Check sheet for the modelled part. Datum: model origin and axes. Units: mm. Face numbers are marked on the shaded views. A direction names the side the tool comes from. Round coordinates to 2 decimals unless told otherwise and drop trailing zeros. Write each loop counter-clockwise with the first axis right and the second up, starting at its lowest first coordinate (ties: lowest second). Pieces come first, ordered by that corner, then holes. Notation, with made-up numbers: (57.5, 32) - (61.5, 32) arc R29 ccw to (61.5, 61) - close; hole circle Ø1 at (-34.75, 61). An arc over 180 degrees is marked (long way). Answer as a JSON object with one key per item and string values. Group by question number.
Item 1: Thickness scan on line 1 (Z direction, x = 69, y = 6.75); line 2 (X direction, y = 5.75, z = -8); line 3 (X direction, y = 0.5, z = 5.5). Record the ranges inside material, lowest first.
Item 2: Set-up check for the marked faces 1, 2, 3 and 4: record each of +Z, -Z, +X, -X, +Y, -Y from which the full face is reachable in a straight line by a thin tool's end or side.
Item 3: Sectioned sample at D-D on z = -32. Record the boundary of the cut face in (x, y), plus the area to 3 significant figures.
Item 4: Sectioned sample at C-C on y = 1.5. Count the separate pieces of the cut face and the enclosed holes in it, plus the area to 3 significant figures.
Item 5: Gauge pin test, flat ends, axial feed: P1, Ø4.5, axis at x = 73.5, z = 5.5, coming from the +Y side; P2, Ø4, axis at x = 60, y = 3.5, coming from the +Z side; P3, Ø2, axis at y = 3, z = 17, coming from the -X side; P4, Ø3.5, axis at x = 90.01, z = -24.99, coming from the +Y side. Record the tip position at first contact, or that the pin passes through.
Item 6: Sectioned sample at B-B on x = 60. Record the boundary of the cut face in (y, z), plus the area to 3 significant figures.
Item 7: Sectioned sample at A-A on z = 16. Record the boundary of the cut face in (x, y), plus the area to 3 significant figures.
Item 8: Release check for a two-part mould opening along Z. For the marked faces 5, 6 and 7 record: pulls with the +Z half, pulls with the -Z half, needs draft (parallel to the pull), parting line crosses it, or undercut.
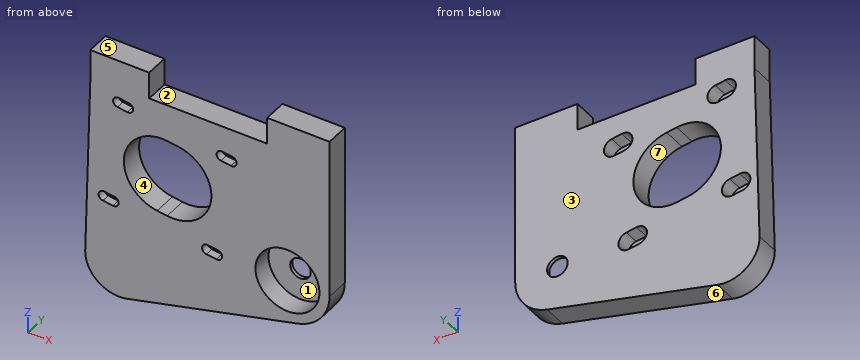
```python
from build123d import *

# Parameters (mm, degrees)
SKETCH2_R           = 3.05
BOSS_EXTRUDE1_DEPTH = 7
SKETCH2_7_R         = 9.5
SKETCH2_7_R_2       = 3.05
CUT_EXTRUDE1_DEPTH  = 6
CUT_EXTRUDE2_START  = 7
CUT_EXTRUDE2_DEPTH  = 4.5


with BuildPart() as part:
    # Sketch2 → Boss-Extrude1 (new body)
    with BuildSketch(Plane(origin=(0, 0, 0), x_dir=(1, 0, 0), z_dir=(0, 1, 0))):
        with BuildLine():
            Line((102.512048312, 24.992099408), (102.512048312, -23.007900592))
            Line((102.512048312, -23.007900592), (84.012048312, -23.007900592))
            Line((84.012048312, -23.007900592), (84.012048312, -15.007900592))
            Line((84.012048312, -15.007900592), (49.012048312, -15.007900592))
            Line((49.012048312, -15.007900592), (49.012048312, -23.007900592))
            Line((49.012048312, -23.007900592), (31.512048312, -23.007900592))
            Line((31.512048312, -23.007900592), (31.512048312, -13.007900592))
            Line((31.512048312, -13.007900592), (30.016072392, 39.708435169))
            ThreePointArc((30.016072392, 39.708435169), (33.741164308, 47.78158038), (42.423514406, 49.696986387))
            Line((42.423514406, 49.696986387), (93.026380929, 37.123208132))
            ThreePointArc((93.026380929, 37.123208132), (99.859107713, 32.691802074), (102.512048312, 24.992099408))
        make_face()
        with Locations(Location((90.012048312, 24.992099408, 0), (0, 0, 270))):
            Circle(SKETCH2_R, mode=Mode.SUBTRACT)
        with BuildLine():
            Line((51.378851017, 18.833843692), (54.349655223, 19.251362995))
            ThreePointArc((54.349655223, 19.251362995), (67.338228674, 9.463770865), (57.550636545, -3.524802586))
            Line((57.550636545, -3.524802586), (54.579832339, -3.942321889))
            ThreePointArc((54.579832339, -3.942321889), (41.591258887, 5.84527024), (51.378851017, 18.833843692))
        make_face(mode=Mode.SUBTRACT)
        with BuildLine():
            Line((65.962554027, 26.437501135), (68.933358233, 26.855020438))
            ThreePointArc((68.933358233, 26.855020438), (70.627519988, 25.578377986), (69.350877536, 23.884216232))
            Line((69.350877536, 23.884216232), (66.38007333, 23.466696929))
            ThreePointArc((66.38007333, 23.466696929), (64.685911575, 24.74333938), (65.962554027, 26.437501135))
        make_face(mode=Mode.SUBTRACT)
        with BuildLine():
            Line((70.694439459, -7.231613202), (73.665243666, -6.814093899))
            ThreePointArc((73.665243666, -6.814093899), (74.941886117, -5.119932145), (73.247724363, -3.843289693))
            Line((73.247724363, -3.843289693), (70.276920157, -4.260808996))
            ThreePointArc((70.276920157, -4.260808996), (69.000277705, -5.954970751), (70.694439459, -7.231613202))
        make_face(mode=Mode.SUBTRACT)
        with BuildLine():
            Line((42.966933535, -11.128460029), (39.996129329, -11.545979332))
            ThreePointArc((39.996129329, -11.545979332), (38.301967574, -10.26933688), (39.578610026, -8.575175126))
            Line((39.578610026, -8.575175126), (42.549414232, -8.157655823))
            ThreePointArc((42.549414232, -8.157655823), (44.243575986, -9.434298275), (42.966933535, -11.128460029))
        make_face(mode=Mode.SUBTRACT)
        with BuildLine():
            Line((38.235048102, 22.540654308), (35.264243896, 22.123135005))
            ThreePointArc((35.264243896, 22.123135005), (33.987601444, 20.428973251), (35.681763199, 19.152330799))
            Line((35.681763199, 19.152330799), (38.652567405, 19.569850102))
            ThreePointArc((38.652567405, 19.569850102), (39.929209857, 21.264011856), (38.235048102, 22.540654308))
        make_face(mode=Mode.SUBTRACT)
    extrude(amount=BOSS_EXTRUDE1_DEPTH)

    # Sketch2<7> → Cut-Extrude1 (cut)
    with BuildSketch(Plane(origin=(0, 0, 0), x_dir=(1, 0, 0), z_dir=(0, 1, 0))):
        with Locations(Location((90.012048312, 24.992099408, 0), (0, 0, 270))):
            Circle(SKETCH2_7_R)
        with Locations(Location((90.012048312, 24.992099408, 0), (0, 0, 270))):
            Circle(SKETCH2_7_R_2, mode=Mode.SUBTRACT)
    extrude(amount=CUT_EXTRUDE1_DEPTH, mode=Mode.SUBTRACT)

    # Sketch2<8> → Cut-Extrude2 (cut)
    with BuildSketch(Plane(origin=(0, 0, 0), x_dir=(1, 0, 0), z_dir=(0, 1, 0)).offset(CUT_EXTRUDE2_START)):
        with BuildLine():
            Line((65.788587651, 27.675336221), (68.759391857, 28.092855524))
            ThreePointArc((68.759391857, 28.092855524), (71.865355074, 25.752344362), (69.524843912, 22.646381146))
            Line((69.524843912, 22.646381146), (66.554039706, 22.228861843))
            ThreePointArc((66.554039706, 22.228861843), (63.448076489, 24.569373004), (65.788587651, 27.675336221))
        make_face()
        with BuildLine():
            Line((70.868405836, -8.469448288), (73.839210042, -8.051928985))
            ThreePointArc((73.839210042, -8.051928985), (76.179721203, -4.945965769), (73.073757987, -2.605454607))
            Line((73.073757987, -2.605454607), (70.10295378, -3.02297391))
            ThreePointArc((70.10295378, -3.02297391), (67.762442619, -6.128937127), (70.868405836, -8.469448288))
        make_face()
        with BuildLine():
            Line((38.061081726, 23.778489394), (35.09027752, 23.360970091))
            ThreePointArc((35.09027752, 23.360970091), (32.749766358, 20.255006874), (35.855729575, 17.914495713))
            Line((35.855729575, 17.914495713), (38.826533781, 18.332015016))
            ThreePointArc((38.826533781, 18.332015016), (41.167044943, 21.437978232), (38.061081726, 23.778489394))
        make_face()
        with BuildLine():
            Line((42.375447856, -6.919820737), (39.404643649, -7.33734004))
            ThreePointArc((39.404643649, -7.33734004), (37.064132488, -10.443303257), (40.170095705, -12.783814418))
            Line((40.170095705, -12.783814418), (43.140899911, -12.366295115))
            ThreePointArc((43.140899911, -12.366295115), (45.481411072, -9.260331898), (42.375447856, -6.919820737))
        make_face()
    extrude(amount=-CUT_EXTRUDE2_DEPTH, mode=Mode.SUBTRACT)


solid = part.part
```
Completed:
{
 "1": {"line 1": "-43.09 to -28.12, -22.57 to 3.43, 8.06 to 15.01", "line 2": "30.92 to 41.49, 67.45 to 102.51", "line 3": "31.3 to 69.01, 74.95 to 102.51"},
 "2": {"face 1": "-Y", "face 2": "+Z, +Y, -Y", "face 3": "+Z, -Z, +X, -X, +Y", "face 4": "+Y, -Y"},
 "3": {"outline": "(30.23, 0) - (83.6, 0) - (83.6, 6) - (96.43, 6) - (96.43, 0) - (100.36, 0) - (100.36, 7) - (30.23, 7) - close", "area": "414 mm²"},
 "4": {"separate pieces": "1", "enclosed holes": "6", "area": "3,620 mm²"},
 "5": {"P1": "y = 2.5", "P2": "z = 15.01", "P3": "x = 31.51", "P4": "through"},
 "6": {"outline": "(0, -45.33) - (7, -45.33) - (7, -18.63) - (0, -18.63) - close; (0, 2.9) - (7, 2.9) - (7, 15.01) - (0, 15.01) - close", "area": "272 mm²"},
 "7": {"outline": "(31.51, 0) - (49.01, 0) - (49.01, 7) - (31.51, 7) - close; (84.01, 0) - (102.51, 0) - (102.51, 7) - (84.01, 7) - close", "area": "252 mm²"},
 "8": {"face 5": "pulls with the +Z half", "face 6": "pulls with the -Z half", "face 7": "undercut"}
}
